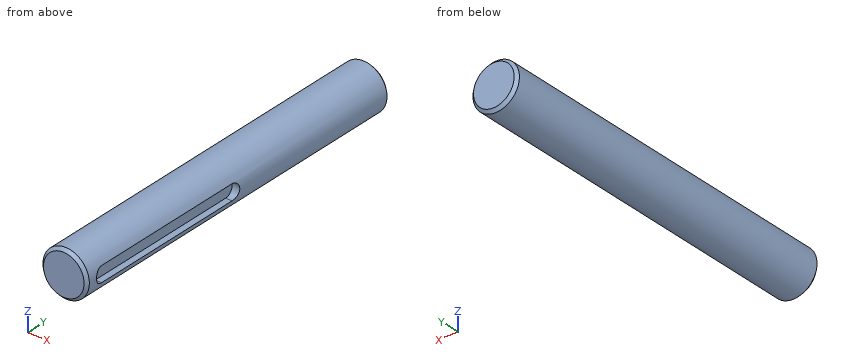
from build123d import *

# Parameters (mm, degrees)
SKETCH1_R           = 12
BOSS_EXTRUDE1_DEPTH = 190
CUT_EXTRUDE1_DEPTH  = 4
CHAMFER1_SIZE       = 1.5


with BuildPart() as part:
    # Sketch1 → Boss-Extrude1 (new body)
    with BuildSketch(Plane(origin=(0, 0, 0), x_dir=(1, 0, 0), z_dir=(0, 1, 0))):
        Circle(SKETCH1_R)
    extrude(amount=BOSS_EXTRUDE1_DEPTH)

    # Sketch2 → Cut-Extrude1 (cut)
    with BuildSketch(Plane(origin=(12, 0, 0), x_dir=(0, 0, -1), z_dir=(1, 0, 0))):
        with BuildLine():
            Line((4, 92), (4, 10))
            ThreePointArc((4, 10), (0, 6), (-4, 10))
            Line((-4, 10), (-4, 92))
            ThreePointArc((-4, 92), (0, 96), (4, 92))
        make_face()
    extrude(amount=-CUT_EXTRUDE1_DEPTH, mode=Mode.SUBTRACT)

    # Chamfer1
    chamfer1_edges = [part.edges().sort_by_distance(p)[0] for p in [
        (-12, 0, 0),
        (-12, 190, 0),
    ]]
    chamfer(chamfer1_edges, length=CHAMFER1_SIZE)


solid = part.part
CAD build for the part. Positions are in the model's coordinates, mm. Round coordinates to 2 decimals unless told otherwise and drop trailing zeros. Write each loop counter-clockwise with the first axis right and the second up, starting at its lowest first coordinate (ties: lowest second). Pieces come first, ordered by that corner, then holes.
(1) Slice it at A-A, the plane z = 0. Write the cut outline in (x, y), and give its area (3 significant figures).
(2) Drop flat-ended pins along their axis: P1, Ø2, axis at y = 142.5, z = 6, coming from the -X side; P2, Ø6, axis at x = 6, y = 118.5, coming from the +Z side; P3, Ø1, axis at x = -6.5, y = 95, coming from the +Z side; P4, Ø12, axis at y = 62, z = 3, coming from the -X side. Give the stop position or say it passes through.
(3) Slice it at B-B, the plane y = 56.5. Write the cut outline in (x, z), and give its area (3 significant figures).
(4) Probe line 1 along Z through (x, y) = (-7, 28); line 2 along X through (y, z) = (121, -10.75); line 3 along X through (y, z) = (42.5, 2.75). List the from-to ranges inside material, lowest first.
(5) Slice it at C-C, the plane y = 147.5. Write the cut outline in (x, z).
From the geometry:
1. outline: (-12, 1.5) - (-10.5, 0) - (10.5, 0) - (12, 1.5) - (12, 6) - (8, 6) - (8, 96) - (12, 96) - (12, 188.5) - (10.5, 190) - (-10.5, 190) - (-12, 188.5) - close
1. area: 4,200 mm2
2. P1: stops at x = -10.91
2. P2: stops at z = 11.62
2. P3: stops at z = 10.39
2. P4: stops at x = -12
3. outline: (8, -4) - (8, 4) - (11.31, 4) arc R12 ccw (long way) to (11.31, -4) - close
3. area: 422 mm2
4. line 1: z = -9.75 to 9.75
4. line 2: x = -5.33 to 5.33
4. line 3: x = -11.68 to 8
5. outline: circle Ø24 at (0, 0)
